Verification items for this drawing (mm, ordinates from the low corner). Give positions to 0.01 mm unless a question says otherwise; leave off trailing zeros. Write each loop counter-clockwise with the first axis right and the second up, starting at its lowest first coordinate (ties: lowest second). Pieces come first, ordered by that corner, then holes. Notation, with made-up numbers: M 65.25,34 L 86.25,34 A22 ccw 86.25,43 Z; hole C -3.5,84 d7. An arc over 180 degrees is marked long. Write each question's results on one line, items separated by ' | '.
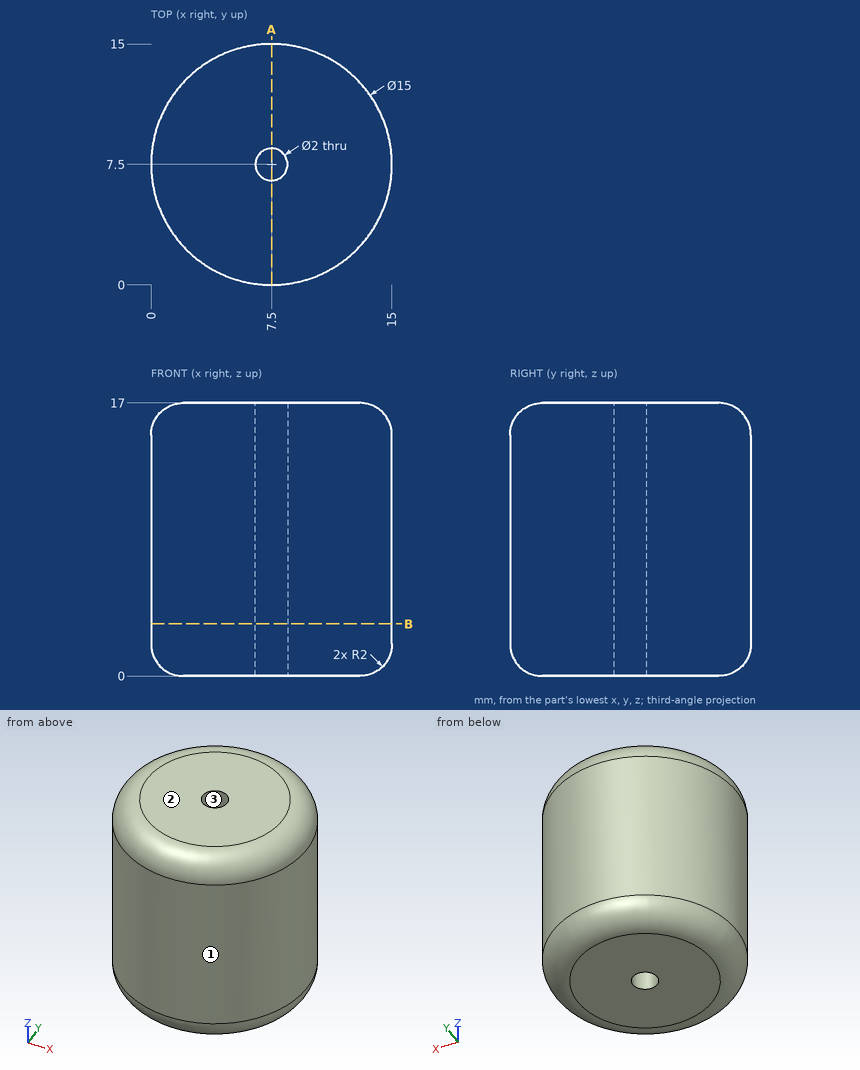
Q1. Depth check by flat-ended pin: P1, Ø5, axis at x = 6, z = 5.5, coming from the +Y side; P2, Ø5, axis at x = 11, z = 5, coming from the -Y side; P3, Ø1, axis at x = 2, y = 4, coming from the -Z side; P4, Ø1.5, axis at x = 4.5, z = 5, coming from the -Y side. Enter the tip coordinate at first touch or a pass-through.
Answer key:
P1: stops at y = 15 | P2: stops at y = 0.07 | P3: stops at z = 0.07 | P4: stops at y = 0.35
Q2. Section check A-A (x = 7.5). Enter the section's corners in (y, z), then the cut area to 3 significant figures.
Answer key:
outline: M 0,2 A2 ccw 2,0 L 6.5,0 L 6.5,17 L 2,17 A2 ccw 0,15 Z; M 8.5,0 L 13,0 A2 ccw 15,2 L 15,15 A2 ccw 13,17 L 8.5,17 Z | area: 218 mm2
Q3. Section check B-B (z = 3.25). Enter the section's corners in (x, y).
Answer key:
outline: C 7.5,7.5 d15; hole C 7.5,7.5 d2
Q4. Release check for a two-part mould opening along Y. For the marked faces 1, 2 and 3 record: released by +Y, released by -Y, zero draft, split by the parting line, or undercut.
Answer key:
face 1: split by the parting line | face 2: zero draft | face 3: undercut
Q5. Material ranges on probe 1 along Y at (x, z) = (7.5, 6.75); probe 2 along Z at (x, y) = (2.25, 5.5); probe 3 along X at (y, z) = (8, 9.25), recorded low to high. Write a range as [from, to].
Answer key:
probe 1: y = [0, 6.5], [8.5, 15] | probe 2: z = [0, 17] | probe 3: x = [0.02, 6.63], [8.37, 14.98]
